Part model, mm, in its own coordinate system. Face numbers are marked on the shaded views. A direction names the side the tool comes from. Round coordinates to 2 decimals unless told otherwise and drop trailing zeros. Loops run counter-clockwise (first coordinate to the right, second up) from the corner with the lowest first, then second, coordinate; pieces in that order, holes last. Notation, with made-up numbers: (-40, 34) -> (19, 34) arc R30 cw to (19, 69) -> close; hole circle Ø2 at (27, 22). An arc over 180 degrees is marked (long way). Use a Markdown table: item, result. Add a question column.
Item 1: Probe line 1 (Y direction, x = 0, z = 76.5) (3 decimals); line 2 (X direction, y = 0, z = 75.5) (3 decimals); line 3 (Z direction, x = -4, y = 17). List the from-to ranges inside material, lowest first. Write a range as [from, to].
Item 2: Cut at D-D, the plane x = -7. List the corners of the cut face in (y, z), plus the area to 3 significant figures.
Item 3: Cut at A-A, the plane z = 55. List the corners of the cut face in (x, y).
Item 4: Flat gauge pins, fed straight in: pin 1 (1.5 mm diameter, centred on x = 7, z = 67, fed in from -Y); pin 2 (11 mm diameter, centred on y = 5.5, z = 70, fed in from -X); pin 3 (10 mm diameter, centred on y = 9, z = 30, fed in from -X). Where does each tip first touch, or does it go through?
Item 5: Cut at B-B, the plane x = 9. List the corners of the cut face in (y, z).
Item 6: Which spindle directions (+Z, -Z, +X, -X, +Y, -Y) get a long thin tool onto all of the face, cutting with end or side? Do the marked faces 1, 2 and 3. Say none if no direction does.
Item 7: Cut at C-C, the plane z = 68. List the corners of the cut face in (x, y).
```python
from build123d import *

# Parameters (mm, degrees)
F0_R     = 19.05
F1_DEPTH = 76.2
F2_R     = 12.7
F3_DEPTH = 9.398
F5_DEPTH = 19.304
F7_D     = 6.35
F7_DEPTH = 12.7
F7_TIP   = 1.9077324654


with BuildPart() as f1:
    # F0 (on Top) → F1 (new body)
    with BuildSketch(Plane.XY):
        Circle(F0_R)
    extrude(amount=F1_DEPTH)

    # F2 (on face) → F3 (join)
    with BuildSketch(Plane.XY.offset(76.2)):
        Circle(F2_R)
    extrude(amount=F3_DEPTH)

    # F4 (on face) → F5 (cut)
    with BuildSketch(Plane.XY.offset(85.598)):
        with BuildLine():
            Line((-15.0368, -12.6474779099), (-15.0368, 12.6474779099))
            ThreePointArc((-15.0368, 12.6474779099), (-19.6485127102, 0), (-15.0368, -12.6474779099))
        make_face()
    extrude(amount=-F5_DEPTH, mode=Mode.SUBTRACT)

    # F7
    with Locations(Plane.XY.offset(85.598)):
        with Locations((0, 0)):
            Hole(F7_D / 2, depth=F7_DEPTH)
            with Locations((0, 0, -(F7_DEPTH + F7_TIP / 2))):  # 118° drill point
                Cone(0, F7_D / 2, F7_TIP, mode=Mode.SUBTRACT)


solid = f1.part
```
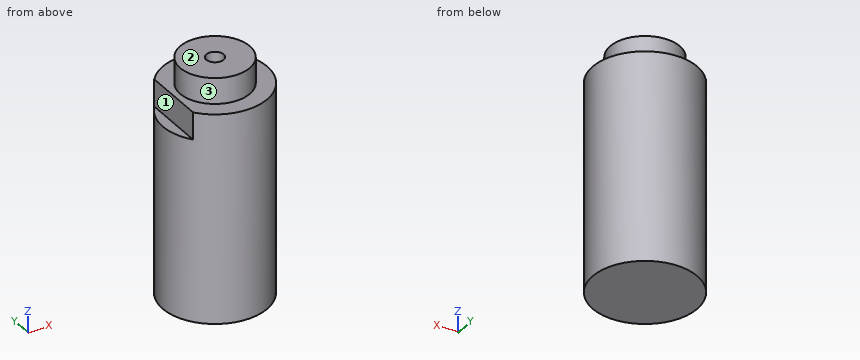
A:
| question | item | result |
|---|---|---|
| 1 | line 1 | y = [-12.7, -3.175], [3.175, 12.7] |
| 1 | line 2 | x = [-15.037, -3.175], [3.175, 19.05] |
| 1 | line 3 | z = [0, 76.2] |
| 2 | outline | (-17.72, 0) -> (17.72, 0) -> (17.72, 76.2) -> (10.6, 76.2) -> (10.6, 85.6) -> (-10.6, 85.6) -> (-10.6, 76.2) -> (-17.72, 76.2) -> close |
| 2 | area | 2,900 mm^2 |
| 3 | outline | circle Ø38.1 at (0, 0) |
| 4 | pin 1 | stops at y = -18 |
| 4 | pin 2 | stops at x = -19 |
| 4 | pin 3 | stops at x = -18.63 |
| 5 | outline | (-16.79, 0) -> (16.79, 0) -> (16.79, 76.2) -> (8.96, 76.2) -> (8.96, 85.6) -> (-8.96, 85.6) -> (-8.96, 76.2) -> (-16.79, 76.2) -> close |
| 6 | face 1 | +Z, -X, +Y, -Y |
| 6 | face 2 | +Z, +X, -X, +Y, -Y |
| 6 | face 3 | +Z |
| 7 | outline | (-15.04, -11.7) arc R19.05 ccw (long way) to (-15.04, 11.7) -> close |
